Could you check a few things on this model? Use its own coordinates, in mm. Face numbers are marked on the shaded views. Coordinates: 2 decimals unless noted, no trailing zeros. Order: outer loops, then holes, each group sorted by start corner. A loop starts at its lowest first (then second) coordinate and runs counter-clockwise, first axis right, second up. Notation, with made-up numbers: M 10.25,77 L 63.25,77 A31 ccw 63.25,103 Z; hole C -1,-14 d5. An arc over 180 degrees is marked long. Write item = value, one per line. Start each with the question number.
from build123d import *

# Parameters (mm, degrees)
F0_W      = 80.264
F0_H      = 101.6
F1_DEPTH  = 6.35
F2_W      = 54.737
F2_H      = 4.7625
F3_DEPTH  = 88.9
F5_DEPTH  = 5.08
F6_W      = 54.737
F6_H      = 3.81
F7_DEPTH  = 88.9
F8_R      = 3.81
F10_D     = 3.048
F10_DEPTH = 9.525
F10_TIP   = 0.9157115834
F12_D     = 3.048
F12_DEPTH = 9.525
F12_TIP   = 0.9157115834
F14_D     = 3.048
F14_DEPTH = 9.525
F14_TIP   = 0.9157115834
F16_D     = 3.048
F16_DEPTH = 9.525
F16_TIP   = 0.9157115834


with BuildPart() as f1:
    # F0 (on Front) → F1 (new body, symmetric)
    with BuildSketch(Plane.XZ):
        Rectangle(F0_W, F0_H)
    extrude(amount=F1_DEPTH, both=True)

    # F2 (on face) → F3 (cut)
    with BuildSketch(Plane.XY.offset(50.8)):
        with Locations((0, -2.69875)):
            Rectangle(F2_W, F2_H)
    extrude(amount=-F3_DEPTH, mode=Mode.SUBTRACT)

    # F4 (on face) → F5 (cut)
    with BuildSketch(Plane.XZ.offset(6.35)):
        with BuildLine():
            add(Edge.make_bspline(
                [(0, -21.021893248), (19.8113411297, -21.021893248), (9.9056705649, 10.510946624), (0, 42.0437864959), (-9.9056705649, 10.510946624), (-19.8113411297, -21.021893248), (0, -21.021893248)],
                knots=[0, 0, 0, 2.0943951024, 2.0943951024, 4.1887902048, 4.1887902048, 6.2831853072, 6.2831853072, 6.2831853072], degree=2, weights=[1, 0.5, 1, 0.5, 1, 0.5, 1]))
        make_face()
    extrude(amount=-F5_DEPTH, mode=Mode.SUBTRACT)

    # F6 (on face) → F7 (cut)
    with BuildSketch(Plane.XY.offset(50.8)):
        with Locations((0, 2.9844999377)):
            Rectangle(F6_W, F6_H)
    extrude(amount=-F7_DEPTH, mode=Mode.SUBTRACT)

    # F8
    f8_edges = [f1.edges().sort_by_distance(p)[0] for p in [
        (40.132, 0, 50.8),
        (-40.132, 0, 50.8),
        (-40.132, 0, -50.8),
        (40.132, 0, -50.8),
    ]]
    fillet(f8_edges, radius=F8_R)

    # F10
    with Locations(Plane(origin=(-40.132, 0, 0), x_dir=(0, -1, 0), z_dir=(-1, 0, 0))):
        with Locations((0, 42.3520989716)):
            Hole(F10_D / 2, depth=F10_DEPTH)
            with Locations((0, 0, -(F10_DEPTH + F10_TIP / 2))):  # 118° drill point
                Cone(0, F10_D / 2, F10_TIP, mode=Mode.SUBTRACT)

    # F12
    with Locations(Plane.YZ.offset(40.132)):
        with Locations((0, 42.3520989716)):
            Hole(F12_D / 2, depth=F12_DEPTH)
            with Locations((0, 0, -(F12_DEPTH + F12_TIP / 2))):  # 118° drill point
                Cone(0, F12_D / 2, F12_TIP, mode=Mode.SUBTRACT)

    # F14
    with Locations(Plane(origin=(0, 6.35, 0), x_dir=(-1, 0, 0), z_dir=(0, 1, 0))):
        with Locations((-36.322, 46.99), (36.322, 46.99), (-36.322, -46.99), (36.322, -46.99)):
            Hole(F14_D / 2, depth=F14_DEPTH)
            with Locations((0, 0, -(F14_DEPTH + F14_TIP / 2))):  # 118° drill point
                Cone(0, F14_D / 2, F14_TIP, mode=Mode.SUBTRACT)

    # F16
    with Locations(Plane.XZ.offset(6.35)):
        with Locations((-35.5702526867, 36.9295366108), (-35.5702526867, -38.6124029756), (36.322, -38.6124029756), (36.322, 36.9295366108)):
            Hole(F16_D / 2, depth=F16_DEPTH)
            with Locations((0, 0, -(F16_DEPTH + F16_TIP / 2))):  # 118° drill point
                Cone(0, F16_D / 2, F16_TIP, mode=Mode.SUBTRACT)


solid = f1.part
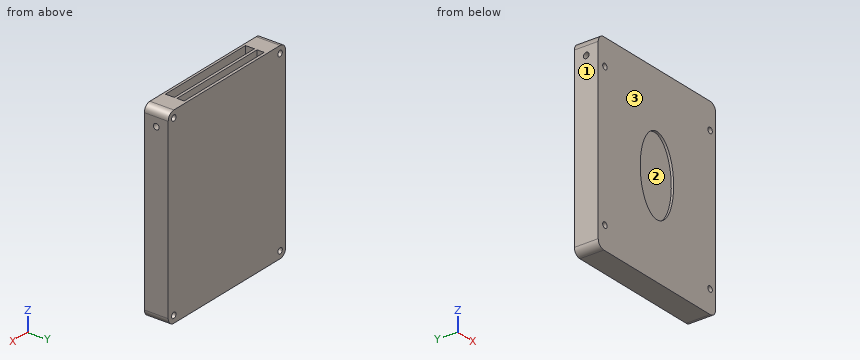
(1) Will these pins go through, and if not, where does the flat tip stop? P1, Ø2.5, axis at y = 0, z = 42.35, coming from the -X side; P2, Ø4, axis at x = 36.32, z = 36.93, coming from the -Y side; P3, Ø1.9, axis at x = -6, y = 2.5, coming from the +Z side.
(2) Thinking about a two-plate mould opening in Y: for the marked faces 1, 2 and 3, which applies, released by +Y, released by -Y, zero draft, split by the parting line, or undercut?
(3) Imagine slicing it at A-A on z = -28.5. List the corners of the cut face in (x, y) for me, plus the area to 3 significant figures.
(4) Imagine slicing it at B-B on x = -18. List the corners of the cut face in (y, z) for me, plus the area to 3 significant figures.
(5) Please list where these lines run through material, in increasing order: probe 1 along Y at (x, z) = (-26, -1.5); probe 2 along X at (y, z) = (0.5, 46.99); probe 3 along X at (y, z) = (2.75, -37). Write a range as from..to.
Response:
q1.P1 = -30.44
q1.P2 = -6.35
q1.P3 = -38.1
q2.face_1 = zero draft
q2.face_2 = undercut
q2.face_3 = released by -Y
q3.outline = M -40.13,-6.35 L 40.13,-6.35 L 40.13,6.35 L -40.13,6.35 Z; hole M -27.37,-5.08 L 27.37,-5.08 L 27.37,-0.32 L -27.37,-0.32 Z; hole M -27.37,1.08 L 27.37,1.08 L 27.37,4.89 L -27.37,4.89 Z
q3.area = 550 mm2
q4.outline = M -6.35,-50.8 L 6.35,-50.8 L 6.35,50.8 L 4.89,50.8 L 4.89,-38.1 L 1.08,-38.1 L 1.08,50.8 L -0.32,50.8 L -0.32,-38.1 L -5.08,-38.1 L -5.08,50.8 L -6.35,50.8 Z
q4.area = 528 mm2
q5.probe_1 = -6.35..-5.08, -0.32..1.08, 4.89..6.35
q5.probe_2 = -40.13..-37.85, -34.8..34.8, 37.85..40.13
q5.probe_3 = -40.13..-27.37, 27.37..40.13
